Could you check a few things on this model? Use its own coordinates, in mm. Face numbers are marked on the shaded views. A direction names the side the tool comes from. Coordinates: 2 decimals unless noted, no trailing zeros. Order: outer loops, then holes, each group sorted by start corner. A loop starts at its lowest first (then second) coordinate and runs counter-clockwise, first axis right, second up. Notation, with made-up numbers: (25, 54) - (66, 54) arc R12 ccw to (66, 75) - close; hole circle Ø3 at (52.25, 51). An arc over 180 degrees is marked (long way). One line per item, written item: value. Start each with the question number.
from build123d import *

# Parameters (mm, degrees)
SKETCH1_W                                       = 15
SKETCH1_H                                       = 30
BOSS_EXTRUDE1_DEPTH                             = 4
BOSS_EXTRUDE2_DEPTH                             = 14
SKETCH3_R                                       = 2.3
CUT_EXTRUDE1_DEPTH                              = 8
CSK_FOR_M3_FLAT_HEAD_MACHINE_SCREW1_D           = 3.4
CSK_FOR_M3_FLAT_HEAD_MACHINE_SCREW1_DEPTH       = 6.35
CSK_FOR_M3_FLAT_HEAD_MACHINE_SCREW1_CSINK_D     = 6.3
CSK_FOR_M3_FLAT_HEAD_MACHINE_SCREW1_CSINK_ANGLE = 90
CSK_FOR_M3_FLAT_HEAD_MACHINE_SCREW1_TIP         = 1.021463052


with BuildPart() as part:
    # Sketch1 → Boss-Extrude1 (new body)
    with BuildSketch(Plane(origin=(0, 0, 0), x_dir=(0, 0, -1), z_dir=(1, 0, 0))):
        with BuildLine():
            Line((-33.857008974, 10.235870452), (-45.565370995, 0.232449935))
            ThreePointArc((-45.565370995, 0.232449935), (-27.604171468, -10.061381798), (-7.5, -15))
            Line((-7.5, -15), (-7.5, 0.096693129))
            ThreePointArc((-7.5, 0.096693129), (-21.290873092, 3.574416464), (-33.857008974, 10.235870452))
        make_face()
        Rectangle(SKETCH1_W, SKETCH1_H)
        with BuildLine():
            Line((-41.931432124, 16.989065709), (-52.538033842, 6.382463992))
            ThreePointArc((-52.538033842, 6.382463992), (-49.147992618, 3.198286628), (-45.565370995, 0.232449935))
            Line((-45.565370995, 0.232449935), (-33.857008974, 10.235870452))
            ThreePointArc((-33.857008974, 10.235870452), (-38.044360457, 13.432954073), (-41.931432124, 16.989065709))
        make_face()
    extrude(amount=BOSS_EXTRUDE1_DEPTH)

    # Sketch2 → Boss-Extrude2 (add)
    with BuildSketch(Plane(origin=(4, 0, 0), x_dir=(0, 0, -1), z_dir=(1, 0, 0))):
        with BuildLine():
            Line((-33.854727787, 10.234284113), (-45.563203072, 0.230766826))
            ThreePointArc((-45.563203072, 0.230766826), (-41.349722145, -2.810292527), (-36.933994133, -5.549418231))
            Line((-36.933994133, -5.549418231), (-24.61890521, 4.97237918))
            ThreePointArc((-24.61890521, 4.97237918), (-29.354954434, 7.395973089), (-33.854727787, 10.234284113))
        make_face()
    extrude(amount=BOSS_EXTRUDE2_DEPTH)

    # Sketch3 → Cut-Extrude1 (cut)
    with BuildSketch(Plane(origin=(4, 0, 0), x_dir=(0, 0, -1), z_dir=(1, 0, 0))):
        with Locations((-39.70896543, 5.232525469)):
            Circle(SKETCH3_R)
    extrude(amount=CUT_EXTRUDE1_DEPTH, mode=Mode.SUBTRACT)

    # CSK for M3 Flat Head Machine Screw1
    with Locations(Plane(origin=(4, 0, 0), x_dir=(0, 0, -1), z_dir=(1, 0, 0))):
        with Locations((-42.74343682, 7.59), (-17.289112213, -5.603347362), (0, 0)):
            CounterSinkHole(CSK_FOR_M3_FLAT_HEAD_MACHINE_SCREW1_D / 2, CSK_FOR_M3_FLAT_HEAD_MACHINE_SCREW1_CSINK_D / 2, depth=CSK_FOR_M3_FLAT_HEAD_MACHINE_SCREW1_DEPTH, counter_sink_angle=CSK_FOR_M3_FLAT_HEAD_MACHINE_SCREW1_CSINK_ANGLE)
            with Locations((0, 0, -(CSK_FOR_M3_FLAT_HEAD_MACHINE_SCREW1_DEPTH + CSK_FOR_M3_FLAT_HEAD_MACHINE_SCREW1_TIP / 2))):  # 118° drill point
                Cone(0, CSK_FOR_M3_FLAT_HEAD_MACHINE_SCREW1_D / 2, CSK_FOR_M3_FLAT_HEAD_MACHINE_SCREW1_TIP, mode=Mode.SUBTRACT)


solid = part.part
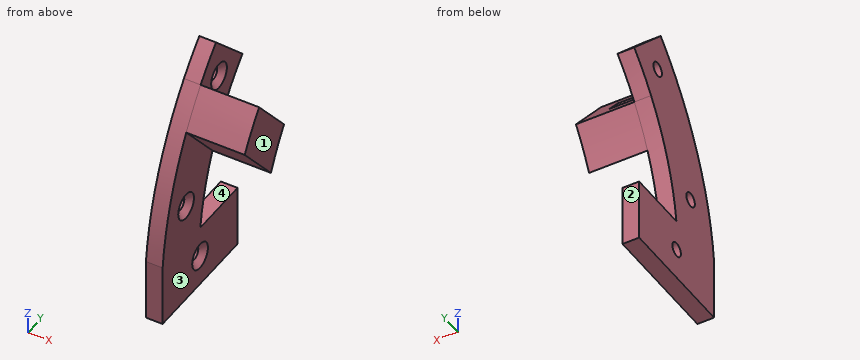
Q1. I'm going to push flat-ended pins straight in: pin 1 (5.5 mm diameter, centred on y = 0, z = 0, fed in from +X); pin 2 (1.2 mm diameter, centred on x = 2, y = 8, fed in from +Z); pin 3 (1 mm diameter, centred on y = 4, z = 2.5, fed in from +X). Where does each tip first touch, or does it pass through?
Q2. I want a section at B-B on y = 7.59. Please give me the cut outline in (x, z).
Q3. I want a section at C-C on x = 5.25. Please give me the cut outline in (y, z), then the cut area to 3 significant figures.
Q4. Which directions (+Z, -Z, +X, -X, +Y, -Y) give clear straight access to the entire face, cutting with the end or side of a thin tool? Please do the marked faces 1, 2, 3 and 4.
Q5. I want a section at A-A on z = 0. Please give me the cut outline in (x, y), then the cut area to 3 significant figures.
Q6. If I drill on L1, parallel to Z at x = 1.4, y = 7.59; L2, parallel to X at y = 11, z = -1; L3, parallel to Z at x = 1.7, y = 0, over which ranges is the centre line in solid material (lowest first)?
Q7. I want a section at D-D on x = 13. Please give me the cut outline in (y, z), then the cut area to 3 significant figures.
Values follow:
1. pin 1: stops at x = 3.6
1. pin 2: stops at z = 51.52
1. pin 3: stops at x = 4
2. outline: (0, -7.5) - (4, -7.5) - (4, 7.5) - (0, 7.5) - close; (0, 29.69) - (18, 29.69) - (18, 36.95) - (4, 36.95) - (4, 39.59) - (2.55, 41.04) - (0, 41.04) - close; (0, 44.44) - (2.55, 44.44) - (4, 45.89) - (4, 51.33) - (0, 51.33) - close
3. outline: (-5.55, 36.93) - (4.97, 24.62) arc R59.3 cw to (10.23, 33.85) - (6.73, 37.96) arc R2.3 cw to (3.74, 41.46) - (0.23, 45.56) arc R74.3 ccw to start
3. area: 149 mm^2
4. face 1: +Z, -Z, +X, +Y, -Y
4. face 2: -Z, +X, -X, +Y
4. face 3: -Z, +X, -Y
4. face 4: +X, -X, +Y
5. outline: (0, -15) - (4, -15) - (4, -3.15) - (2.55, -1.7) - (0, -1.7) - close; (0, 1.7) - (2.55, 1.7) - (4, 3.15) - (4, 15) - (0, 15) - close
5. area: 104 mm^2
6. L1: z = -7.5 to 7.5, 29.69 to 41.04, 44.44 to 51.33
6. L2: x = 0 to 4
6. L3: z = -7.5 to -1.7, 1.7 to 45.26
7. outline: (-5.55, 36.93) - (4.97, 24.62) arc R59.3 cw to (10.23, 33.85) - (0.23, 45.56) arc R74.3 ccw to start
7. area: 158 mm^2
